Autodesk Fusion 360 part; units mm, degrees
sketch "Base" plane through (0, 0, 0) normal (0, 0, 1) x (1, 0, 0)
  circle A0 centre (0, 0) radius 30
  circle A1 centre (0, 0) radius 28
  dimension "d1" = 60
  dimension "d2" = 56
extrude "Extrude1" add sketch "Base" along normal blind 2 contours A1 makes body 1
extrude "Extrude2" add sketch "Base" along normal blind 113 bodies 1
sketch "Sketch2" plane through (0, 0, 0) normal (0, 0, 1) x (1, 0, 0)
  circle A0 centre (0, 0) radius 28
  line L0 (0, -2) -> (27.9285, -2)
  line L1 (-27.9285, -2) -> (0, -2)
  line L2 (0, 2) -> (-27.9285, 2)
  line L3 (27.9285, 2) -> (0, 2)
  circle A1 centre (0, 0) radius 30
extrude "Extrude3" add sketch "Sketch2" along normal blind 3 separate body makes body 2
extrude "Extrude4" add sketch "Sketch2" along normal blind 5 contours A0 L0 L1 bodies 2
extrude "Extrude5" add sketch "Sketch2" along normal blind 5 contours A0 L2 L3 bodies 2
extrude "Extrude6" add sketch "Sketch2" along normal blind 110 contours A0 L0 L1 L2 L3 bodies 2
sketch "Sketch6" plane through (0, 2, 0) normal (0, 1, 0) x (-1, 0, 0)
  line L0 (-27.9285, 5) -> (27.9285, 5)
  line L1 (27.9285, 5) -> (27.9285, 110)
  line L2 (27.9285, 110) -> (-27.9285, 110)
  line L3 (-27.9285, 110) -> (-27.9285, 5)
  line L4 (-2.5, 7.5) -> (2.5, 7.5)
  line L5 (2.5, 7.5) -> (2.5, 110)
  line L6 (-2.5, 110) -> (2.5, 110)
  line L7 (-2.5, 110) -> (-2.5, 7.5)
  dimension "d15" = 102.5
  dimension "d16" = 5
extrude "Extrude7" cut sketch "Sketch6" against normal blind 4 contours L2 L4 L5 L6 L7 bodies 2
hidden bodies 1
Work out the finished part from the listing and answer in its coordinate system (mm). A direction names the side the tool comes from. Coordinates: 2 decimals unless noted, no trailing zeros. Loops run counter-clockwise (first coordinate to the right, second up) from the corner with the lowest first, then second, coordinate; pieces in that order, holes last.
1) Flat-ended cylindrical pins translate along their axes: pin 1 (10 mm diameter, centred on x = -20.5, z = 35, fed in from +Y); pin 2 (2 mm diameter, centred on x = -21.5, z = 72.5, fed in from -Y); pin 3 (2 mm diameter, centred on x = -1, y = 0.5, fed in from +Z). Find the tip coordinate at first contact, or state that the pin passes through.
Results:
pin 1: stops at y = 2
pin 2: stops at y = -2
pin 3: stops at z = 7.5
2) Section B-B (z = 90) is taken. Give the vertices of the cut face in (x, y).
Results:
outline: (-27.93, -2) - (-2.5, -2) - (-2.5, 2) - (-27.93, 2) arc R28 ccw to start; (2.5, -2) - (27.93, -2) arc R28 ccw to (27.93, 2) - (2.5, 2) - close
3) For faces 4 (the flat face through (0, 0, 0)), 5 (the cylindrical face through (-29.97, -1.32, 1.48)), 6 (the flat face through (-2.5, 0, 58)), 7 (the flat face through (0, -12, 5)), 8 (the flat face through (0, 12, 5)), determine the directions among +Z, -Z, +X, -X, +Y, -Y from which every point of the face is accessible in a straight line to the end or side of a thin tool.
Results:
face 4: -Z, +X, -X, +Y, -Y
face 5: +Z, -Z
face 6: +Z, +Y, -Y
face 7: +Z, +X, -X, -Y
face 8: +Z, +X, -X, +Y
4) Section A-A (y = 0) is taken. Give the vertices of the cut face in (x, z), plus the area to 3 significant figures.
Results:
outline: (-30, 0) - (30, 0) - (30, 3) - (28, 3) - (28, 110) - (2.5, 110) - (2.5, 7.5) - (-2.5, 7.5) - (-2.5, 110) - (-28, 110) - (-28, 3) - (-30, 3) - close
area: 5,660 mm2
5) Section C-C (x = 0) is taken. Give the vertices of the cut face in (y, z), plus the area to 3 significant figures.
Results:
outline: (-30, 0) - (30, 0) - (30, 3) - (28, 3) - (28, 5) - (2, 5) - (2, 7.5) - (-2, 7.5) - (-2, 5) - (-28, 5) - (-28, 3) - (-30, 3) - close
area: 302 mm2
6) Consider probe 1 along Y at (x, z) = (-4.5, 49); probe 2 along Z at (x, y) = (-16.5, 5). Determine where each line is inside the solid, lowest interval first.
Results:
probe 1: y = -2 to 2
probe 2: z = 0 to 5
7) For a pull along X with two mould halves and no side action, classify faces 1 (the flat face through (0, 0, 7.5)), 2 (the cylindrical face through (-28, 0, 32)), 3 (the flat face through (-25, 13, 3)) as +X half, -X half, draft (parallel to the pull), parting line (faces both ways), or undercut.
Results:
face 1: undercut
face 2: parting line
face 3: draft
8) Section D-D (y = 17) is taken. Give the vertices of the cut face in (x, z), plus the area to 3 significant figures.
Results:
outline: (-24.72, 0) - (24.72, 0) - (24.72, 3) - (22.25, 3) - (22.25, 5) - (-22.25, 5) - (-22.25, 3) - (-24.72, 3) - close
area: 237 mm2
